```python
from build123d import *

# Parameters (mm, degrees)
SKETCH1_R           = 1.6
BOSS_EXTRUDE1_DEPTH = 8
CHAMFER1_SIZE       = 1
SKETCH2_R           = 1.6
BOSS_EXTRUDE3_DEPTH = 8
FILLET1_R           = 10
CHAMFER2_SIZE       = 1
CHAMFER3_SIZE       = 1
CHAMFER4_SIZE       = 1
SKETCH3_R           = 1.6
BOSS_EXTRUDE4_DEPTH = 8
CHAMFER5_SIZE       = 1
FILLET2_R           = 10


with BuildPart() as part:
    # Sketch1 → Boss-Extrude1 (new body)
    with BuildSketch(Plane.XY):
        with BuildLine():
            Line((-0.5, 3), (60.5, 3))
            ThreePointArc((60.5, 3), (62.267766953, 2.267766953), (63, 0.5))
            Line((63, 0.5), (63, -0.5))
            ThreePointArc((63, -0.5), (62.267766953, -2.267766953), (60.5, -3))
            Line((60.5, -3), (-0.5, -3))
            ThreePointArc((-0.5, -3), (-2.267766953, -2.267766953), (-3, -0.5))
            Line((-3, -0.5), (-3, 0.5))
            ThreePointArc((-3, 0.5), (-2.267766953, 2.267766953), (-0.5, 3))
        make_face()
        Circle(SKETCH1_R, mode=Mode.SUBTRACT)
        with Locations((7.5, 0)):
            Circle(SKETCH1_R, mode=Mode.SUBTRACT)
        with Locations((15, 0)):
            Circle(SKETCH1_R, mode=Mode.SUBTRACT)
        with Locations((22.5, 0)):
            Circle(SKETCH1_R, mode=Mode.SUBTRACT)
        with Locations((30, 0)):
            Circle(SKETCH1_R, mode=Mode.SUBTRACT)
        with Locations((37.5, 0)):
            Circle(SKETCH1_R, mode=Mode.SUBTRACT)
        with Locations((45, 0)):
            Circle(SKETCH1_R, mode=Mode.SUBTRACT)
        with Locations((52.5, 0)):
            Circle(SKETCH1_R, mode=Mode.SUBTRACT)
        with Locations((60, 0)):
            Circle(SKETCH1_R, mode=Mode.SUBTRACT)
    extrude(amount=BOSS_EXTRUDE1_DEPTH)

    # Chamfer1
    chamfer1_edges = [part.edges().sort_by_distance(p)[0] for p in [
        (-1.6, 0, 0),
        (-1.6, 0, 8),
        (5.9, 0, 0),
        (5.9, 0, 8),
        (13.4, 0, 0),
        (13.4, 0, 8),
        (20.9, 0, 0),
        (20.9, 0, 8),
        (28.4, 0, 0),
        (28.4, 0, 8),
    ]]
    chamfer(chamfer1_edges, length=CHAMFER1_SIZE)

    # Sketch2 → Boss-Extrude3 (add)
    with BuildSketch(Plane.XY.offset(8)):
        with BuildLine():
            ThreePointArc((-3, 0.5), (-2.809698831, 1.456708581), (-2.267766953, 2.267766953))
            Line((-2.267766953, 2.267766953), (-18.529200529, -13.993666623))
            ThreePointArc((-18.529200529, -13.993666623), (-19.261433576, -15.761433576), (-18.529200529, -17.529200529))
            Line((-18.529200529, -17.529200529), (-17.822093748, -18.23630731))
            ThreePointArc((-17.822093748, -18.23630731), (-16.054326795, -18.968540357), (-14.286559842, -18.23630731))
            Line((-14.286559842, -18.23630731), (0.949747468, -3))
            Line((0.949747468, -3), (-0.5, -3))
            ThreePointArc((-0.5, -3), (-2.267766953, -2.267766953), (-3, -0.5))
            Line((-3, -0.5), (-3, 0.5))
        make_face()
        with Locations((-16.054326795, -15.761433576)):
            Circle(SKETCH2_R, mode=Mode.SUBTRACT)
        with Locations((-10.751025936, -10.458132717)):
            Circle(SKETCH2_R, mode=Mode.SUBTRACT)
        with Locations((-5.447725077, -5.154831858)):
            Circle(SKETCH2_R, mode=Mode.SUBTRACT)
    extrude(amount=-BOSS_EXTRUDE3_DEPTH)

    # Fillet1
    fillet1_edges = [part.edges().sort_by_distance(p)[0] for p in [
        (0.949747468, -3, 4),
    ]]
    fillet(fillet1_edges, radius=FILLET1_R)

    # Chamfer2
    chamfer2_edges = [part.edges().sort_by_distance(p)[0] for p in [
        (-17.654326795, -15.761433576, 0),
        (-17.654326795, -15.761433576, 8),
        (-12.351025936, -10.458132717, 8),
        (-7.047725077, -5.154831858, 8),
        (-7.047725077, -5.154831858, 0),
        (-12.351025936, -10.458132717, 0),
    ]]
    chamfer(chamfer2_edges, length=CHAMFER2_SIZE)

    # Chamfer3
    chamfer3_edges = [part.edges().sort_by_distance(p)[0] for p in [
        (35.9, 0, 0),
        (35.9, 0, 8),
        (43.4, 0, 0),
        (43.4, 0, 8),
    ]]
    chamfer(chamfer3_edges, length=CHAMFER3_SIZE)

    # Chamfer4
    chamfer4_edges = [part.edges().sort_by_distance(p)[0] for p in [
        (50.9, 0, 0),
        (50.9, 0, 8),
        (58.4, 0, 0),
        (58.4, 0, 8),
    ]]
    chamfer(chamfer4_edges, length=CHAMFER4_SIZE)

    # Sketch3 → Boss-Extrude4 (add)
    with BuildSketch(Plane.XY.offset(8)):
        with BuildLine():
            ThreePointArc((-18.529200529, -17.529200529), (-19.071132407, -16.718142157), (-19.261433576, -15.761433576))
            Line((-19.261433576, -15.761433576), (-19.261433576, -37.761433576))
            ThreePointArc((-19.261433576, -37.761433576), (-18.529200529, -39.529200529), (-16.761433576, -40.261433576))
            Line((-16.761433576, -40.261433576), (-15.761433576, -40.261433576))
            ThreePointArc((-15.761433576, -40.261433576), (-13.993666623, -39.529200529), (-13.261433576, -37.761433576))
            Line((-13.261433576, -37.761433576), (-13.261433576, -17.211181044))
            Line((-13.261433576, -17.211181044), (-14.286559842, -18.23630731))
            ThreePointArc((-14.286559842, -18.23630731), (-16.054326795, -18.968540357), (-17.822093748, -18.23630731))
            Line((-17.822093748, -18.23630731), (-18.529200529, -17.529200529))
        make_face()
        with Locations((-16.261433576, -30.261433576)):
            Circle(SKETCH3_R, mode=Mode.SUBTRACT)
        with Locations((-16.261433576, -37.261433576)):
            Circle(SKETCH3_R, mode=Mode.SUBTRACT)
        with Locations((-16.261433576, -23.261433576)):
            Circle(SKETCH3_R, mode=Mode.SUBTRACT)
    extrude(amount=-BOSS_EXTRUDE4_DEPTH)

    # Chamfer5
    chamfer5_edges = [part.edges().sort_by_distance(p)[0] for p in [
        (-17.861433576, -37.261433576, 8),
        (-17.861433576, -30.261433576, 8),
        (-17.861433576, -23.261433576, 8),
        (-17.861433576, -23.261433576, 0),
        (-17.861433576, -30.261433576, 0),
        (-17.861433576, -37.261433576, 0),
    ]]
    chamfer(chamfer5_edges, length=CHAMFER5_SIZE)

    # Fillet2
    fillet2_edges = [part.edges().sort_by_distance(p)[0] for p in [
        (-13.261433576, -17.211181044, 4),
    ]]
    fillet(fillet2_edges, radius=FILLET2_R)


solid = part.part
```
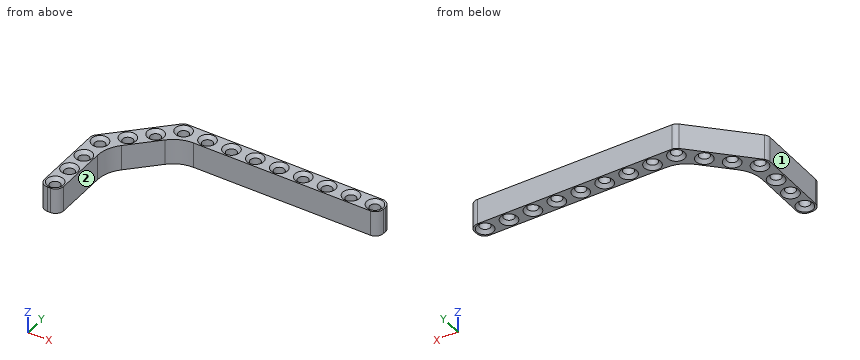
Input: part model. Units: mm. Frame: model coordinates. Face numbers are marked on the shaded views. A direction names the side the tool comes from. Round coordinates to 2 decimals unless told otherwise and drop trailing zeros. Write each loop counter-clockwise with the first axis right and the second up, starting at its lowest first coordinate (ties: lowest second). Pieces come first, ordered by that corner, then holes. Notation, with made-up numbers: (24, -24.5) -> (63, -24.5) arc R25 cw to (63, 4.5) -> close; hole circle Ø1 at (58, -24.5). An arc over 180 degrees is marked (long way). Answer as CSV lines item,"result".
1. Reachability of the marked faces 1 and 2 from +Z, -Z, +X, -X, +Y, -Y: full face, straight path, thin tool, end or side. Return the list, or none.
Geometry says:
face 1,"+Z, -Z, -X, +Y, -Y"
face 2,"+Z, -Z, +X, -Y"
2. Section C-C (x = 11.5). Return the cut outline in (y, z), plus the area to 3 significant figures.
Geometry says:
outline,"(-3, 0) -> (3, 0) -> (3, 8) -> (-3, 8) -> close"
area,"48.0 mm^2"
3. Contact query for flat-ended pins moving along their axis: P1, Ø5, axis at x = -5.45, y = -5.15, coming from the +Z side; P2, Ø3.5, axis at x = 52.5, y = 0, coming from the +Z side; P3, Ø1, axis at x = -2.5, z = 2.5, coming from the -Y side. Output: stop coordinate, or through.
Geometry says:
P1,"stops at z = 7.91"
P2,"stops at z = 7.15"
P3,"stops at y = -6.95"
4. Section B-B (z = 5.5). Give the number of separate pieces and of enclosed holes in the cut face, plus the area to 3 significant figures.
Geometry says:
separate pieces,"1"
enclosed holes,"15"
area,"539 mm^2"
5. Section A-A (x = 22.5). Return the cut outline in (y, z).
Geometry says:
outline,"(-3, 0) -> (-2.6, 0) -> (-1.6, 1) -> (-1.6, 7) -> (-2.6, 8) -> (-3, 8) -> close; (1.6, 1) -> (2.6, 0) -> (3, 0) -> (3, 8) -> (2.6, 8) -> (1.6, 7) -> close"
6. Ray query, L1, parallel to Y at x = 22.5, z = 3.6; L2, parallel to X at y = -27, z = 5; L3, parallel to X at y = -6.5, z = 3.75. Return the intervals inside material, ascending. Write a range as [from, to].
Geometry says:
L1,"y = [-3, -1.6], [1.6, 3]"
L2,"x = [-19.26, -13.26]"
L3,"x = [-11.04, -6.31], [-4.58, -2.55]"
